```python
from build123d import *

# Parameters (mm, degrees)
BOSS_EXTRUDE1_DEPTH            = 14
M3_CLEARANCE_HOLE1_D           = 3.4
M3_CLEARANCE_HOLE1_CSINK_D     = 3.45
M3_CLEARANCE_HOLE1_CSINK_ANGLE = 90
SKETCH2_W                      = 0.61
SKETCH2_H                      = 6.5
CUT_EXTRUDE1_DEPTH             = 23.181073013
M2_TAPPED_HOLE1_D              = 1.6


with BuildPart() as part:
    # Sketch1 → Boss-Extrude1 (new body)
    with BuildSketch(Plane(origin=(0, 0, 0), x_dir=(1, 0, 0), z_dir=(0, 1, 0))):
        Polygon((-10, 0), (0, 0), (0, -14), (-3, -14), (-3, -2), (-10, -2), align=None)
    extrude(amount=BOSS_EXTRUDE1_DEPTH)

    # M3 Clearance Hole1 (through all)
    with Locations(Plane.XY.offset(2)):
        with Locations((-6.5, 10.5), (-6.5, 3.5)):
            CounterSinkHole(M3_CLEARANCE_HOLE1_D / 2, M3_CLEARANCE_HOLE1_CSINK_D / 2, counter_sink_angle=M3_CLEARANCE_HOLE1_CSINK_ANGLE)

    # Sketch2 → Cut-Extrude1 (cut, through all)
    with BuildSketch(Plane.XY.offset(14)):
        with Locations((-0.305, 7)):
            Rectangle(SKETCH2_W, SKETCH2_H)
    extrude(amount=-CUT_EXTRUDE1_DEPTH, mode=Mode.SUBTRACT)

    # M2 Tapped Hole1 (through all)
    with Locations(Plane(origin=(0, 5.858814373, -1.158558045), x_dir=(0, 0, 1), z_dir=(1, 0, 0))):
        with Locations((8.158558045, -6.141185627), (8.158558045, 3.858814373)):
            Hole(M2_TAPPED_HOLE1_D / 2)


solid = part.part
```
Geometry: final body of the model. Coordinates: model frame, mm. A direction names the side the tool comes from. Round coordinates to 2 decimals unless told otherwise and drop trailing zeros. Loops run counter-clockwise (first coordinate to the right, second up) from the corner with the lowest first, then second, coordinate; pieces in that order, holes last. Notation, with made-up numbers: (67.5, 77.25) -> (85.5, 77.25) arc R4 ccw to (85.5, 84.25) -> close; hole circle Ø10 at (-5, -40). An arc over 180 degrees is marked (long way). Write each question's results on one line, items separated by ' | '.
Item 1: Pin query (flat end, axial travel): pin 1 Ø1.4 at (y, z) = (2, 7) entering from -X (1 decimal); pin 2 Ø1 at (x, y) = (-6, 2) entering from +Z. Return the tip coordinate at first contact, or that it passes through.
Answers below:
pin 1: passes through | pin 2: stops at z = 2
Item 2: Cut plane A-A on x = -6.5. Return the cut outline in (y, z) (3 decimals).
Answers below:
outline: (0, 0) -> (1.8, 0) -> (1.8, 1.975) -> (1.775, 2) -> (0, 2) -> close; (5.2, 0) -> (8.8, 0) -> (8.8, 1.975) -> (8.775, 2) -> (5.225, 2) -> (5.2, 1.975) -> close; (12.2, 0) -> (14, 0) -> (14, 2) -> (12.225, 2) -> (12.2, 1.975) -> close
Item 3: Cut plane C-C on z = 7. Return the cut outline in (x, y), and give its area (3 significant figures).
Answers below:
outline: (-3, 0) -> (0, 0) -> (0, 1.2) -> (-3, 1.2) -> close; (-3, 2.8) -> (0, 2.8) -> (0, 3.75) -> (-0.61, 3.75) -> (-0.61, 10.25) -> (0, 10.25) -> (0, 11.2) -> (-3, 11.2) -> close; (-3, 12.8) -> (0, 12.8) -> (0, 14) -> (-3, 14) -> close | area: 28.4 mm²
Item 4: Pull-direction query (Z, two-part tool) for faces 1 (the face through (-1.5, 2, 7.8)), 2 (the face through (-2.7, 0, 5.3)), 3 (the face through (-5, 7, 0)); classes: pulls with the +Z half, pulls with the -Z half, needs draft (parallel to the pull), parting line crosses it, or undercut.
Answers below:
face 1: undercut | face 2: needs draft | face 3: pulls with the -Z half
Item 5: Cut plane B-B on y = 10.5. Return the cut outline in (x, z) (3 decimals).
Answers below:
outline: (-10, 0) -> (-8.2, 0) -> (-8.2, 1.975) -> (-8.225, 2) -> (-10, 2) -> close; (-4.8, 0) -> (0, 0) -> (0, 14) -> (-3, 14) -> (-3, 2) -> (-4.775, 2) -> (-4.8, 1.975) -> close
Item 6: Cut plane D-D on x = -1.5. Return the cut outline in (y, z).
Answers below:
outline: (0, 0) -> (14, 0) -> (14, 14) -> (0, 14) -> close; hole circle Ø1.6 at (2, 7); hole circle Ø1.6 at (12, 7)
Item 7: Line query: probe 1 along Y at (x, z) = (-0.8, 7); probe 2 along Y at (x, z) = (-6.5, 0.7); probe 3 along X at (y, z) = (3.5, 1). Output: solid intervals per line, ascending. Write a range as [from, to].
Answers below:
probe 1: y = [0, 1.2], [2.8, 11.2], [12.8, 14] | probe 2: y = [0, 1.8], [5.2, 8.8], [12.2, 14] | probe 3: x = [-10, -8.2], [-4.8, 0]
Item 8: Set-up query: faces 4 (the face through (-3, 7, 8)), 5 (the face through (-0.61, 7, 7)), 6 (the face through (-1.5, 12, 7.8)). Return all of +Z, -Z, +X, -X, +Y, -Y with unobstructed straight access to the full face (end or side cutting, diameter ignored); none if empty.
Answers below:
face 4: +Z, -X, +Y, -Y | face 5: +Z, -Z, +X | face 6: +X, -X
